Can you work these out from the model? Positions are in its coordinate system, mm. A direction names the side the tool comes from. Round coordinates to 2 decimals unless told otherwise and drop trailing zeros.
from build123d import *

# Parameters (mm, degrees)
SKETCH1_W                                   = 160
SKETCH1_H                                   = 160
BOSS_EXTRUDE1_DEPTH                         = 25.4
CBORE_FOR_0_BINDING_HEAD_MACHINE_SC_2_COUNT = 2
CBORE_FOR_0_BINDING_HEAD_MACHINE_SC_2_PITCH = 134.6
CBORE_FOR_0_BINDING_HEAD_MACHINE_SC_3_COUNT = 2
CBORE_FOR_0_BINDING_HEAD_MACHINE_SC_3_PITCH = 190.353145495
CBORE_FOR_0_BINDING_HEAD_MACHINE_SC_4_COUNT = 2
CBORE_FOR_0_BINDING_HEAD_MACHINE_SC_4_PITCH = 134.6


with BuildPart() as part:
    # Sketch1 → Boss-Extrude1 (new body)
    with BuildSketch(Plane(origin=(0, 0, 0), x_dir=(1, 0, 0), z_dir=(0, 1, 0))):
        Rectangle(SKETCH1_W, SKETCH1_H)
    extrude(amount=BOSS_EXTRUDE1_DEPTH)

    # Sketch3 → CBORE for _0 Binding Head Machine Screw1 (revolve, cut)
    with BuildSketch(Plane(origin=(-67.3, 0, -67.3), x_dir=(0, 0, -1), z_dir=(1, 0, 0))):
        Polygon((0, 0), (0, 25.4), (0.80645, 25.4), (0.80645, 0.8128), (1.98501, 0.8128), (1.98501, 0.87249), (2.8575, 0), align=None)
    cbore_for_0_binding_head_machine_screw1 = revolve(axis=Axis((-67.3, -6.35, -67.3), (0, 1, 0)), mode=Mode.SUBTRACT)

    # CBORE for _0 Binding Head Machine Sc 2: CBORE for _0 Binding Head Machine Screw1 ×2
    with Locations(*[(i * CBORE_FOR_0_BINDING_HEAD_MACHINE_SC_2_PITCH, 0, 0) for i in range(1, CBORE_FOR_0_BINDING_HEAD_MACHINE_SC_2_COUNT)]):
        add(cbore_for_0_binding_head_machine_screw1, mode=Mode.SUBTRACT)

    # CBORE for _0 Binding Head Machine Sc 3: CBORE for _0 Binding Head Machine Screw1 ×2
    with Locations(*[Vector(0.707106781, 0, 0.707106781) * (i * CBORE_FOR_0_BINDING_HEAD_MACHINE_SC_3_PITCH) for i in range(1, CBORE_FOR_0_BINDING_HEAD_MACHINE_SC_3_COUNT)]):
        add(cbore_for_0_binding_head_machine_screw1, mode=Mode.SUBTRACT)

    # CBORE for _0 Binding Head Machine Sc 4: CBORE for _0 Binding Head Machine Screw1 ×2
    with Locations(*[(0, 0, i * CBORE_FOR_0_BINDING_HEAD_MACHINE_SC_4_PITCH) for i in range(1, CBORE_FOR_0_BINDING_HEAD_MACHINE_SC_4_COUNT)]):
        add(cbore_for_0_binding_head_machine_screw1, mode=Mode.SUBTRACT)


solid = part.part
(1) If I drill on line 1 (X direction, y = 17.75, z = -67.3), over which ranges is the centre line in solid material (lowest first)?
Worked answers:
line 1: x = -80 to -68.11, -66.49 to 66.49, 68.11 to 80
(2) For faces 4 (the flat face through (-1, 25.4, -1)), 5 (the flat face through (-66, 0.813, 67)), which set-ups out of +Z, -Z, +X, -X, +Y, -Y let a thin tool reach every point of the face, with its end or its side?
Worked answers:
face 4: +Z, -Z, +X, -X, +Y
face 5: -Y
(3) If we mould it in two halves opening along X, with no side actions, what happens to faces 1 (the flat face through (-67, 0.813, -66)), 2 (the flat face through (80, 13, 1)), 3 (the flat face through (-1, 13, -80))? For each: released by +X, released by -X, zero draft, split by the parting line, or undercut.
Worked answers:
face 1: undercut
face 2: released by +X
face 3: zero draft
(4) Will these pins go through, and if not, where does the flat tip stop? P1, Ø1.2, axis at x = 67.5, z = -67.5, coming from the -Y side; P2, Ø2.5, axis at x = -67.3, z = -67.3, coming from the +Y side; P3, Ø4.5, axis at x = -67.5, z = -67.5, coming from the -Y side.
Worked answers:
P1: stops at y = 0.81
P2: stops at y = 25.4
P3: stops at y = 0.32
